```python
from build123d import *

# Parameters (mm, degrees)
F0_W      = 330.2
F0_H      = 228.6
F1_DEPTH  = 76.2
F4_W      = 287.104944
F4_H      = 158.488579
F5_DEPTH  = 127
F2_R      = 25.4
F6_DEPTH  = 76.2
F6_FACE_R = 25.4
F7_DEPTH  = 152.4


with BuildPart() as f1:
    # F0 (on Top) → F1 (new body)
    with BuildSketch(Plane.XY):
        with Locations((17.809838, 37.883661)):
            Rectangle(F0_W, F0_H)
    extrude(amount=F1_DEPTH)

    # F4 (on face) → F5 (cut)
    with BuildSketch(Plane.XY.offset(76.2)):
        with Locations((9.872635, 38.312387)):
            Rectangle(F4_W, F4_H)
    extrude(amount=-F5_DEPTH, mode=Mode.SUBTRACT)

    # F2 (on face) → F6 (join)
    with BuildSketch(Plane(origin=(0, 152.183661, 0), x_dir=(-1, 0, 0), z_dir=(0, 1, 0))):
        with Locations((-146.609987, 40.1991)):
            Circle(F2_R)
        with Locations((-58.958468, 42.370036)):
            Circle(F2_R)
        with Locations((13.496502, 43.998241)):
            Circle(F2_R)
        with Locations((91.650177, 45.897806)):
            Circle(F2_R)
    extrude(amount=F6_DEPTH)

    # F6_face (on face) → F7 (cut)
    with BuildSketch(Plane(origin=(146.609987, 228.383661, 40.1991), x_dir=(-1, 0, 0), z_dir=(0, 1, 0))):
        Circle(F6_FACE_R)
        with Locations((87.651519, 2.170936)):
            Circle(F6_FACE_R)
        with Locations((160.106489, 3.799141)):
            Circle(F6_FACE_R)
        with Locations((238.260164, 5.698706)):
            Circle(F6_FACE_R)
    extrude(amount=-F7_DEPTH, mode=Mode.SUBTRACT)


solid = f1.part
```
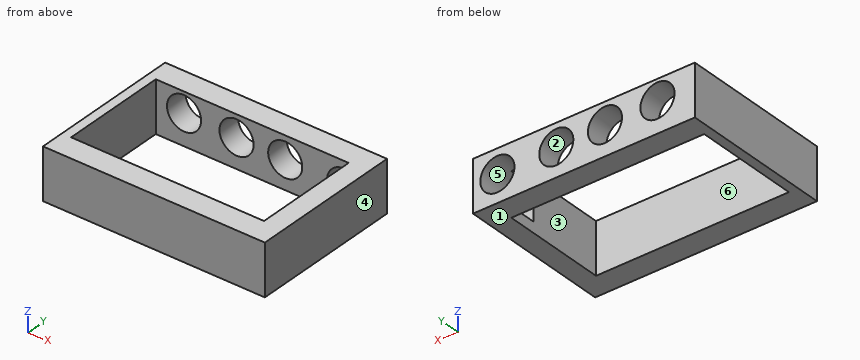
The model under review builds one solid part; all positions refer to its coordinate system, in mm. Face numbers are marked on the shaded views. A direction names the side the tool comes from. Give positions to 0.01 mm unless a question says otherwise; leave off trailing zeros. Write each loop counter-clockwise with the first axis right and the second up, starting at its lowest first coordinate (ties: lowest second). Pieces come first, ordered by that corner, then holes. Notation, with made-up numbers: (68.5, -21) -> (89.5, -21) arc R33 ccw to (89.5, 15) -> close; hole circle Ø11 at (22.25, 87.5). An arc over 180 degrees is marked (long way). Put each result on its own line as item: value.
(1) For pin 1 Ø20.5 at (x, z) = (165, 32) entering from +Y, flat-tipped, find the tip position at first contact; note if it passes through.
Results are:
pin 1: y = 152.18
(2) We need section D-D, the plane z = 26.5. Give the boundary of the cut face in (x, y).
Results are:
outline: (-147.29, -76.42) -> (182.91, -76.42) -> (182.91, 152.18) -> (168, 152.18) -> (168, 75.98) -> (153.43, 75.98) -> (153.43, -40.93) -> (-133.68, -40.93) -> (-133.68, 117.56) -> (-108.05, 117.56) -> (-108.05, 152.18) -> (-147.29, 152.18) -> close; (-75.25, 117.56) -> (-31.91, 117.56) -> (-31.91, 152.18) -> (-75.25, 152.18) -> close; (4.91, 117.56) -> (39.13, 117.56) -> (39.13, 152.18) -> (4.91, 152.18) -> close; (78.79, 117.56) -> (125.22, 117.56) -> (125.22, 152.18) -> (78.79, 152.18) -> close
(3) Tool access review of the marked faces 4, 5 and 6: name each direction out of +Z, -Z, +X, -X, +Y, -Y from which nothing blocks a thin tool from reaching the whole face with its end or side.
Results are:
face 4: +Z, -Z, +X, +Y, -Y
face 5: +Y
face 6: +Z, -Z
(4) We need section B-B, the plane z = 8. Give the boundary of the cut face in (x, y).
Results are:
outline: (-147.29, -76.42) -> (182.91, -76.42) -> (182.91, 152.18) -> (-147.29, 152.18) -> close; hole (-133.68, -40.93) -> (153.43, -40.93) -> (153.43, 117.56) -> (-133.68, 117.56) -> close
(5) To check wall thickness, follow probe 1 along Y at (x, z) = (68, 11); probe 2 along X at (y, z) = (51, 48); probe 3 along Y at (x, z) = (154.5, 59). State the ranges of each line that lie inside material, in increasing order. Write a range as from..to.
Results are:
probe 1: -76.42..-40.93, 117.56..152.18
probe 2: -147.29..-133.68, 153.43..182.91
probe 3: -76.42..75.98
(6) We need section A-A, the plane y = 48. Give the boundary of the cut face in (x, z), and give its area (3 significant figures).
Results are:
outline: (-147.29, 0) -> (-133.68, 0) -> (-133.68, 76.2) -> (-147.29, 76.2) -> close; (153.43, 0) -> (182.91, 0) -> (182.91, 76.2) -> (153.43, 76.2) -> close
area: 3,280 mm²
(7) The part is to be moulded in two halves that separate along Z. For the marked faces 1, 2 and 3, say which applies: pulls with the +Z half, pulls with the -Z half, needs draft (parallel to the pull), parting line crosses it, or undercut.
Results are:
face 1: pulls with the -Z half
face 2: undercut
face 3: needs draft
(8) We need section C-C, the plane x = 24.5. Give the boundary of the cut face in (y, z).
Results are:
outline: (-76.42, 0) -> (-40.93, 0) -> (-40.93, 76.2) -> (-76.42, 76.2) -> close; (117.56, 0) -> (152.18, 0) -> (152.18, 76.2) -> (117.56, 76.2) -> close
